Geometry: final body of the model. Coordinates: model frame, mm. A direction names the side the tool comes from. Coordinates: 2 decimals unless noted, no trailing zeros. Order: outer loops, then holes, each group sorted by start corner. A loop starts at its lowest first (then second) coordinate and runs counter-clockwise, first axis right, second up. Notation, with made-up numbers: (24.5, 49) - (47.5, 49) arc R24 ccw to (47.5, 66) - close; hole circle Ø3 at (70, 77.5). An arc over 180 degrees is marked (long way). Use a Markdown table: item, result. Add a question column.
```python
from build123d import *

# Parameters (mm, degrees)
F1_DEPTH = 431.8
F3_DEPTH = 57.151
F4_W     = 12.7
F4_H     = 38.1
F4_W_2   = 6.35
F5_DEPTH = 57.151


# Not quite as in the source:
# - ends of sketch curves that miss each other by under 0.0002 mm in the source are joined


with BuildPart() as f1:
    # F0 (on Top) → F1 (new body)
    with BuildSketch(Plane.XY):
        with BuildLine():
            ThreePointArc((0, 12.7), (3.7197438789, 3.7197438789), (12.7, 0))
            Line((12.7, 0), (15.9004, 0))
            ThreePointArc((15.9004, 0), (18.127503518, 0.922496482), (19.05, 3.1496))
            Line((19.05, 3.1496), (19.05, 34.9504))
            ThreePointArc((19.05, 34.9504), (18.127503518, 37.177503518), (15.9004, 38.1))
            Line((15.9004, 38.1), (3.1496, 38.1))
            ThreePointArc((3.1496, 38.1), (0.922496482, 37.177503518), (0, 34.9504))
            Line((0, 34.9504), (0, 12.7))
        make_face()
        with BuildLine():
            Line((19.05, 34.9504), (19.05, 3.1496))
            ThreePointArc((19.05, 3.1496), (19.972496482, 0.922496482), (22.1996, 0))
            Line((22.1996, 0), (34.9504, 0))
            ThreePointArc((34.9504, 0), (37.177503518, 0.922496482), (38.1, 3.1496))
            Line((38.1, 3.1496), (38.1, 34.9504))
            ThreePointArc((38.1, 34.9504), (37.177503518, 37.177503518), (34.9504, 38.1))
            Line((34.9504, 38.1), (22.1996, 38.1))
            ThreePointArc((22.1996, 38.1), (19.972496482, 37.177503518), (19.05, 34.9504))
        make_face()
        with BuildLine():
            Line((38.1, 34.9504), (38.1, 3.1496))
            ThreePointArc((38.1, 3.1496), (39.022496482, 0.922496482), (41.2496, 0))
            Line((41.2496, 0), (44.45, 0))
            ThreePointArc((44.45, 0), (53.4302561211, 3.7197438789), (57.15, 12.7))
            Line((57.15, 12.7), (57.15, 34.9504))
            ThreePointArc((57.15, 34.9504), (56.227503518, 37.177503518), (54.0004, 38.1))
            Line((54.0004, 38.1), (41.2496, 38.1))
            ThreePointArc((41.2496, 38.1), (39.022496482, 37.177503518), (38.1, 34.9504))
        make_face()
        with BuildLine():
            ThreePointArc((19.0499988437, 41.2496), (19.9724953256, 39.022496482), (22.1995988437, 38.1))
            Line((22.1995988437, 38.1), (34.9504, 38.1))
            Line((34.9504, 38.1), (41.2496, 38.1))
            Line((41.2496, 38.1), (54.0004, 38.1))
            ThreePointArc((54.0004, 38.1), (56.2275023617, 39.022496482), (57.1499988437, 41.2496))
            Line((57.1499988437, 41.2496), (57.1499988437, 44.45))
            ThreePointArc((57.1499988437, 44.45), (53.4302549647, 53.4302561211), (44.4499988437, 57.15))
            Line((44.4499988437, 57.15), (22.1995988437, 57.15))
            ThreePointArc((22.1995988437, 57.15), (19.9724953256, 56.227503518), (19.0499988437, 54.0004))
            Line((19.0499988437, 54.0004), (19.0499988437, 41.2496))
        make_face()
    extrude(amount=F1_DEPTH)

    # F2 (on face) → F3 (cut, through all)
    with BuildSketch(Plane.YZ.offset(57.15)):
        Polygon((57.15, 0), (57.15, 57.15), (0, 0), (12.7, 0), align=None)
        Polygon((12.7, 431.8), (0, 431.8), (57.15, 374.65), (57.15, 431.8), align=None)
    extrude(amount=-F3_DEPTH, mode=Mode.SUBTRACT)

    # F4 (on face) → F5 (cut, through all)
    with BuildSketch(Plane.YZ.offset(57.15)):
        with Locations((6.35, 374.65)):
            Rectangle(F4_W, F4_H)
        with Locations((15.875, 374.65)):
            Rectangle(F4_W_2, F4_H)
    extrude(amount=-F5_DEPTH, mode=Mode.SUBTRACT)


solid = f1.part
```
1) Pin query (flat end, axial travel): pin 1 (5 mm diameter, centred on x = 40.5, y = 37, fed in from +Z); pin 2 (14 mm diameter, centred on x = 10, z = 261.5, fed in from +Y); pin 3 (12 mm diameter, centred on x = 28.5, y = 35.5, fed in from +Z). Return the tip coordinate at first contact, or that it passes through.
2) Section A-A (z = 347). Return loops of the section in (x, y), then the cut area to 3 significant figures.
3) Section B-B (y = 50). Return loops of the section in (x, z), then the cut area to 3 significant figures.
4) Draft query along Z for faces 1 (the face through (3.62, 3.82, 175.31)), 2 (the face through (29, 9, 355.6)), 3 (the face through (29, 29, 29)). Return one class per face: pulls with the +Z half, pulls with the -Z half, needs draft (parallel to the pull), parting line crosses it, or undercut.
5) Set-up query: faces 4 (the face through (29, 28.2, 403.6)), 5 (the face through (10, 38.1, 213)), 6 (the face through (29, 10, 393.7)). Return all of +Z, -Z, +X, -X, +Y, -Y with unobstructed straight access to the full face (end or side cutting, diameter ignored); none if empty.
6) Ray query, line 1 along X through (y, z) = (41, 143.5); line 2 along Y through (x, z) = (55, 181.5); line 3 along Z through (x, y) = (40, 15.5). Return the intervals inside material, ascending.
Values follow:
| question | item | result |
|---|---|---|
| 1 | pin 1 | stops at z = 397.3 |
| 1 | pin 2 | stops at y = 38.1 |
| 1 | pin 3 | stops at z = 402.3 |
| 2 | outline | (0, 12.7) arc R12.7 ccw to (12.7, 0) - (15.9, 0) arc R3.15 ccw to (19.05, 3.15) arc R3.15 ccw to (22.2, 0) - (34.95, 0) arc R3.15 ccw to (38.1, 3.15) arc R3.15 ccw to (41.25, 0) - (44.45, 0) arc R12.7 ccw to (57.15, 12.7) - (57.15, 34.95) arc R3.15 ccw to (54, 38.1) arc R3.15 ccw to (57.15, 41.25) - (57.15, 44.45) arc R12.7 ccw to (44.45, 57.15) - (22.2, 57.15) arc R3.15 ccw to (19.05, 54) - (19.05, 41.25) arc R3.15 ccw to (22.2, 38.1) arc R3.15 ccw to (19.05, 34.95) arc R3.15 ccw to (15.9, 38.1) - (3.15, 38.1) arc R3.15 ccw to (0, 34.95) - close; hole (34.95, 38.1) arc R3.15 cw to (38.1, 34.95) arc R3.15 cw to (41.25, 38.1) - close |
| 2 | area | 2,770 mm² |
| 3 | outline | (19.05, 50) - (55.87, 50) - (55.87, 381.8) - (19.05, 381.8) - close |
| 3 | area | 12,200 mm² |
| 4 | face 1 | needs draft |
| 4 | face 2 | undercut |
| 4 | face 3 | pulls with the -Z half |
| 5 | face 4 | +Z, +X, -X, +Y |
| 5 | face 5 | +Z, -Z, -X, +Y |
| 5 | face 6 | +X, -X, -Y |
| 6 | line 1 | x = 19.06 to 57.14 |
| 6 | line 2 | y = 5.63 to 37.94, 38.26 to 51.52 |
| 6 | line 3 | z = 15.5 to 355.6, 393.7 to 416.3 |
